Check sheet for the modelled part. Datum: model origin and axes. Units: mm. Face numbers are marked on the shaded views. A direction names the side the tool comes from. Coordinates: 2 decimals unless noted, no trailing zeros. Loops run counter-clockwise (first coordinate to the right, second up) from the corner with the lowest first, then second, coordinate; pieces in that order, holes last.
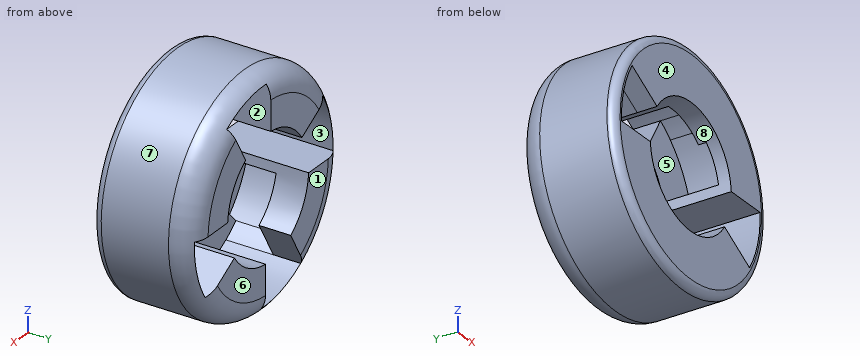
```python
from build123d import *

# Parameters (mm, degrees)
SKETCH2_W          = 6.75
SKETCH2_H          = 12.5
CUT_EXTRUDE1_DEPTH = 10
CIRPATTERN1_COUNT  = 4
CUT_EXTRUDE2_DEPTH = 10
CUT_EXTRUDE3_START = 6
CUT_EXTRUDE3_DEPTH = 7
FILLET1_R          = 3
CUT_EXTRUDE5_START = 6
CUT_EXTRUDE5_DEPTH = 6
CIRPATTERN2_COUNT  = 2
FILLET2_R          = 1


with BuildPart() as part:
    # Sketch2 → Revolve1 (revolve)
    with BuildSketch(Plane(origin=(0, 0, 0), x_dir=(0, 0, -1), z_dir=(1, 0, 0))):
        with Locations((-11.125, 6.25)):
            Rectangle(SKETCH2_W, SKETCH2_H)
    revolve(axis=Axis((0, 31, 0), (0, -1, 0)))

    # Sketch3 → Cut-Extrude1 (cut)
    with BuildSketch(Plane(origin=(0, 12.5, 0), x_dir=(1, 0, 0), z_dir=(0, 1, 0))):
        with BuildLine():
            Line((-7.05329404, 11.216663639), (0.5, -1.866025404))
            Line((0.5, -1.866025404), (0.5, 13.240562677))
            ThreePointArc((0.5, 13.240562677), (-3.429352348, 12.798517198), (-7.05329404, 11.216663639))
        make_face()
    cut_extrude1 = extrude(amount=-CUT_EXTRUDE1_DEPTH, mode=Mode.SUBTRACT)

    # CirPattern1: Cut-Extrude1 ×4 about axis
    cirpattern1_axis = Axis((0, 0, 0), (0, 1, 0))
    for i in range(1, CIRPATTERN1_COUNT):
        add(cut_extrude1.rotate(cirpattern1_axis, i * 360 / CIRPATTERN1_COUNT), mode=Mode.SUBTRACT)

    # Sketch4 → Cut-Extrude2 (cut)
    with BuildSketch(Plane(origin=(0, 2.5, 0), x_dir=(1, 0, 0), z_dir=(0, 1, 0))):
        with BuildLine():
            Line((-7.733854149, 0.5), (-13.240562677, 0.5))
            ThreePointArc((-13.240562677, 0.5), (-12.798517198, -3.429352348), (-11.216663639, -7.05329404))
            Line((-11.216663639, -7.05329404), (-6.447714162, -4.299939776))
            ThreePointArc((-6.447714162, -4.299939776), (-7.485925154, -2.0058476), (-7.733854149, 0.5))
        make_face()
    cut_extrude2 = extrude(amount=-CUT_EXTRUDE2_DEPTH, mode=Mode.SUBTRACT)

    # Sketch5 → Cut-Extrude3 (cut)
    with BuildSketch(Plane(origin=(0, 2.5, 0), x_dir=(1, 0, 0), z_dir=(0, 1, 0)).offset(CUT_EXTRUDE3_START)):
        with BuildLine():
            Line((0, 0), (-8.951570251, 9.768924713))
            ThreePointArc((-8.951570251, 9.768924713), (-11.4748366, 6.625), (-12.935922094, 2.867824885))
            Line((-12.935922094, 2.867824885), (0, 0))
        make_face()
    cut_extrude3 = extrude(amount=-CUT_EXTRUDE3_DEPTH, mode=Mode.SUBTRACT)

    # Fillet1
    # the kernel refuses this fillet: 3 mm, written as the material it takes off along each edge
    with BuildSketch(Plane(origin=(0, 12.5, 0), x_dir=(0, 0, 1), z_dir=(1, 0, 0))) as fillet1_piece_1:
        with BuildLine():
            CenterArc((14.5 - FILLET1_R, FILLET1_R), FILLET1_R, 270, 90)
            Line((14.5 - FILLET1_R, 0), (14.5, 0))
            Line((14.5, 0), (14.5, FILLET1_R))
        make_face()
    revolve(axis=Axis((0, 12.5, 0), (0, -1, 0)), mode=Mode.SUBTRACT)

    # Sketch8 → Cut-Extrude5 (cut)
    with BuildSketch(Plane(origin=(0, 2.5, 0), x_dir=(1, 0, 0), z_dir=(0, 1, 0)).offset(CUT_EXTRUDE5_START)):
        with BuildLine():
            Line((-4.299939776, 6.447714162), (-7.05329404, 11.216663639))
            ThreePointArc((-7.05329404, 11.216663639), (-8.035104682, 10.535634426), (-8.951570251, 9.768924713))
            Line((-8.951570251, 9.768924713), (-5.235824109, 5.71389936))
            ThreePointArc((-5.235824109, 5.71389936), (-4.781978593, 6.098785186), (-4.299939776, 6.447714162))
        make_face()
    cut_extrude5 = extrude(amount=-CUT_EXTRUDE5_DEPTH, mode=Mode.SUBTRACT)

    # CirPattern2: Cut-Extrude2, Cut-Extrude3, Cut-Extrude5 ×2 about axis
    cirpattern2_axis = Axis((0, 0, 0), (0, 1, 0))
    add([cut_extrude2.rotate(cirpattern2_axis, i * 360 / CIRPATTERN2_COUNT) for i in range(1, CIRPATTERN2_COUNT)], mode=Mode.SUBTRACT)
    add([cut_extrude3.rotate(cirpattern2_axis, i * 360 / CIRPATTERN2_COUNT) for i in range(1, CIRPATTERN2_COUNT)], mode=Mode.SUBTRACT)
    add([cut_extrude5.rotate(cirpattern2_axis, i * 360 / CIRPATTERN2_COUNT) for i in range(1, CIRPATTERN2_COUNT)], mode=Mode.SUBTRACT)

    # Fillet2
    fillet2_edges = [part.edges().sort_by_distance(p)[0] for p in [
        (0, 0, -14.5),
    ]]
    fillet(fillet2_edges, radius=FILLET2_R)


solid = part.part
```
1) Section check D-D on x = -12. Give the number of separate pieces and of enclosed holes in the cut face, plus the area to 3 significant figures.
Answer sheet:
separate pieces: 2
enclosed holes: 1
area: 98.2 mm2
2) Set-up check for the marked faces 1, 2, 3, 4 and 5: record each of +Z, -Z, +X, -X, +Y, -Y from which the full face is reachable in a straight line by a thin tool's end or side.
Answer sheet:
face 1: +Z, -Z, +X, -X, +Y
face 2: +Y
face 3: +Y, -Y
face 4: +Z, -Z, +X, -X, -Y
face 5: none
3) Mould release check, pull along Z, two halves, no side actions. Record for the marked faces 6, 7 and 8: +Z half, -Z half, draft (parallel to the pull), parting line (faces both ways), or undercut.
Answer sheet:
face 6: draft
face 7: parting line
face 8: undercut
4) Section check C-C on y = 6.5. Enter the section's corners in (x, z).
Answer sheet:
outline: circle Ø29 at (0, 0); hole (-13.24, -0.5) - (-7.73, -0.5) arc R7.75 ccw to (-7.57, -1.68) - (-12.94, -2.87) arc R13.25 ccw to (0.5, -13.24) - (0.5, -7.73) arc R7.75 ccw to (6.45, -4.3) - (11.22, -7.05) arc R13.25 ccw to (13.24, 0.5) - (7.73, 0.5) arc R7.75 ccw to (7.57, 1.68) - (12.94, 2.87) arc R13.25 ccw to (-0.5, 13.24) - (-0.5, 7.73) arc R7.75 ccw to (-6.45, 4.3) - (-11.22, 7.05) arc R13.25 ccw to start
5) Scan lines: line 1 (Y direction, x = -8.5, z = -8); line 2 (Y direction, x = -6.5, z = -9); line 3 (X direction, y = 11.75, z = 5.5). Record each from-to range of solid material in increasing order.
Answer sheet:
line 1: y = 0 to 1.5, 8.5 to 12.5
line 2: y = 0 to 2.5, 8.5 to 12.5
line 3: x = -12.31 to -12.05, -8.53 to -5.46, 5.46 to 12.31
6) Section check B-B on x = 0. Enter the section's corners in (y, z), plus the area to 3 significant figures.
Answer sheet:
outline: (0, -13.5) arc R1 ccw to (1, -14.5) - (9.5, -14.5) arc R3 ccw to (11.94, -13.25) - (2.5, -13.25) - (2.5, -7.75) - (0, -7.75) - close; (0, 7.75) - (2.5, 7.75) - (2.5, 13.25) - (11.94, 13.25) arc R3 ccw to (9.5, 14.5) - (1, 14.5) arc R1 ccw to (0, 13.5) - close
area: 55.1 mm2
7) Depth check by flat-ended pin: pin 1 (1.5 mm diameter, centred on x = -9, y = 9, fed in from -Z); pin 2 (1 mm diameter, centred on x = -9.5, y = 9.5, fed in from -Z); pin 3 (1.7 mm diameter, centred on y = 7.5, z = -11, fed in from -X). Enter the tip coordinate at first touch or a pass-through.
Answer sheet:
pin 1: stops at z = -11.92
pin 2: stops at z = -11.37
pin 3: stops at x = -10.36
8) Section check A-A on z = 0. Enter the section's corners in (x, y).
Answer sheet:
outline: (-14.5, 1) arc R1 ccw to (-13.5, 0) - (-13.25, 0) - (-13.25, 11.94) arc R3 ccw to (-14.5, 9.5) - close; (13.25, 0) - (13.5, 0) arc R1 ccw to (14.5, 1) - (14.5, 9.5) arc R3 ccw to (13.25, 11.94) - close
